The model under review builds one solid part; all positions refer to its coordinate system, in mm. A direction names the side the tool comes from. Give positions to 0.01 mm unless a question says otherwise; leave off trailing zeros. Order: outer loops, then holes, each group sorted by start corner. A loop starts at its lowest first (then second) coordinate and runs counter-clockwise, first axis right, second up. Notation, with made-up numbers: M 57,-39.5 L 71,-39.5 A19 ccw 71,-13.5 Z; hole C 8.25,-2 d3. An arc over 180 degrees is marked long. One line per question, with ' | ' between items. Start each with the question number.
1. Insertion check: P1, Ø1.1, axis at y = -8, z = 34.5, coming from the +X side; P2, Ø8, axis at x = 6.5, z = 25.5, coming from the +Y side; P3, Ø0.8, axis at y = -11, z = 34.5, coming from the -X side; P4, Ø1.5, axis at x = 27, z = -27, coming from the -Y side. Each pin has a flat end and moves straight along its axis. Give the tip position at first contact, or say it passes through.
2. Wall thickness on L1, parallel to X at y = 1, z = 20; L2, parallel to Z at x = 27, y = -30; L3, parallel to Y at x = 34, z = -20: over which ranges is each line inside the solid? List them lowest first.
3. For faces 4 (the face through (0, 2, -32)), 5 (the face through (-1, -36, 34)), 6 (the face through (-30, 5, 25)), list the 3-axis set-ups (+Z, -Z, +X, -X, +Y, -Y) from which the entire face can be reached by the end or side of a thin tool; tool diameter is ignored.
4. We need section A-A on x = -12. Write out the cut boundary in (y, z), then the cut area to 3 significant figures.
5. We need section D-D on z = -20. Write out the cut boundary in (x, y), then the cut area to 3 significant figures.
6. We need section B-B on y = -28. Write out the cut boundary in (x, z).
7. The part is to be moulded in two halves that separate along Z. For faces 1 (the face through (0, 5, -34)), 2 (the face through (-1, -27, 35)), 3 (the face through (30, 2, -23)), say which applies: +Z half, -Z half, draft (parallel to the pull), parting line (faces both ways), or undercut.
8. We need section C-C on z = -12. Write out the cut boundary in (x, y), then the cut area to 3 significant figures.
```python
from build123d import *

# Parameters (mm, degrees)
SKETCH_1_W          = 80
SKETCH_1_H          = 70
SKETCH_1_R          = 3
SKETCH_1_W_2        = 40
SKETCH_1_H_2        = 64
EXTRUDE_1_DEPTH     = 5
SKETCH_2_W          = 80
SKETCH_2_H          = 1
EXTRUDE_2_DEPTH     = 60
SKETCH_3_W          = 20
SKETCH_3_H          = 22
CUT_EXTRUDE_1_DEPTH = 101.498756211
SKETCH_5_W          = 0.5
SKETCH_5_H          = 70
CUT_EXTRUDE_2_DEPTH = 0.5
SKETCH_6_W          = 80
SKETCH_6_H          = 0.5
CUT_EXTRUDE_3_DEPTH = 0.5


with BuildPart() as part:
    # 草图1 → 凸台-拉伸1 (new body)
    with BuildSketch(Plane(origin=(0, 0, 0), x_dir=(1, 0, 0), z_dir=(0, 1, 0))):
        Rectangle(SKETCH_1_W, SKETCH_1_H)
        with Locations(Location((-30, 20, 0), (0, 0, 270))):
            Circle(SKETCH_1_R, mode=Mode.SUBTRACT)
        with Locations(Location((-30, -20, 0), (0, 0, 270))):
            Circle(SKETCH_1_R, mode=Mode.SUBTRACT)
        with Locations(Location((30, -20, 0), (0, 0, 270))):
            Circle(SKETCH_1_R, mode=Mode.SUBTRACT)
        with Locations(Location((30, 20, 0), (0, 0, 270))):
            Circle(SKETCH_1_R, mode=Mode.SUBTRACT)
        Rectangle(SKETCH_1_W_2, SKETCH_1_H_2, mode=Mode.SUBTRACT)
    extrude(amount=EXTRUDE_1_DEPTH)

    # 草图2 → 凸台-拉伸2 (add)
    with BuildSketch(Plane.XZ):
        with Locations((0, 34.5)):
            Rectangle(SKETCH_2_W, SKETCH_2_H)
        with Locations((0, -34.5)):
            Rectangle(SKETCH_2_W, SKETCH_2_H)
    extrude(amount=EXTRUDE_2_DEPTH)

    # 草图3 → 切除-拉伸1 (cut, through all)
    with BuildSketch(Plane.XY.offset(35)):
        with Locations((30, -11)):
            Rectangle(SKETCH_3_W, SKETCH_3_H)
        with Locations((-30, -11)):
            Rectangle(SKETCH_3_W, SKETCH_3_H)
    extrude(amount=-CUT_EXTRUDE_1_DEPTH, mode=Mode.SUBTRACT)

    # 草图5 → 切除-拉伸2 (cut)
    with BuildSketch(Plane(origin=(0, 5, 0), x_dir=(1, 0, 0), z_dir=(0, 1, 0))):
        with Locations((-19.75, 0)):
            Rectangle(SKETCH_5_W, SKETCH_5_H)
        with Locations((19.75, 0)):
            Rectangle(SKETCH_5_W, SKETCH_5_H)
    extrude(amount=-CUT_EXTRUDE_2_DEPTH, mode=Mode.SUBTRACT)

    # 草图6 → 切除-拉伸3 (cut)
    with BuildSketch(Plane(origin=(0, 5, 0), x_dir=(1, 0, 0), z_dir=(0, 1, 0))):
        with Locations((0, -14.75)):
            Rectangle(SKETCH_6_W, SKETCH_6_H)
        with Locations((0, 14.75)):
            Rectangle(SKETCH_6_W, SKETCH_6_H)
    extrude(amount=-CUT_EXTRUDE_3_DEPTH, mode=Mode.SUBTRACT)


solid = part.part
```
Entries:
1) P1: stops at x = 20 | P2: passes through | P3: stops at x = -20 | P4: stops at y = 0
2) L1: x = -40 to -33, -27 to -20, 20 to 27, 33 to 40 | L2: z = -35 to -34, 34 to 35 | L3: y = 0 to 5
3) face 4: +Y, -Y | face 5: +X, -X, -Y | face 6: +Z, -Z, +X, -X, +Y
4) outline: M -60,-35 L 5,-35 L 5,-32 L 0,-32 L 0,-34 L -60,-34 Z; M -60,34 L 0,34 L 0,32 L 5,32 L 5,35 L -60,35 Z | area: 150 mm^2
5) outline: M -40,0 L -33,0 L -33,5 L -40,5 Z; M -27,0 L -20,0 L -20,5 L -27,5 Z; M 20,0 L 27,0 L 27,5 L 20,5 Z; M 33,0 L 40,0 L 40,5 L 33,5 Z | area: 140 mm^2
6) outline: M -40,-35 L 40,-35 L 40,-34 L -40,-34 Z; M -40,34 L 40,34 L 40,35 L -40,35 Z
7) face 1: draft | face 2: +Z half | face 3: undercut
8) outline: M -40,0 L -20,0 L -20,5 L -40,5 Z; M 20,0 L 40,0 L 40,5 L 20,5 Z | area: 200 mm^2
